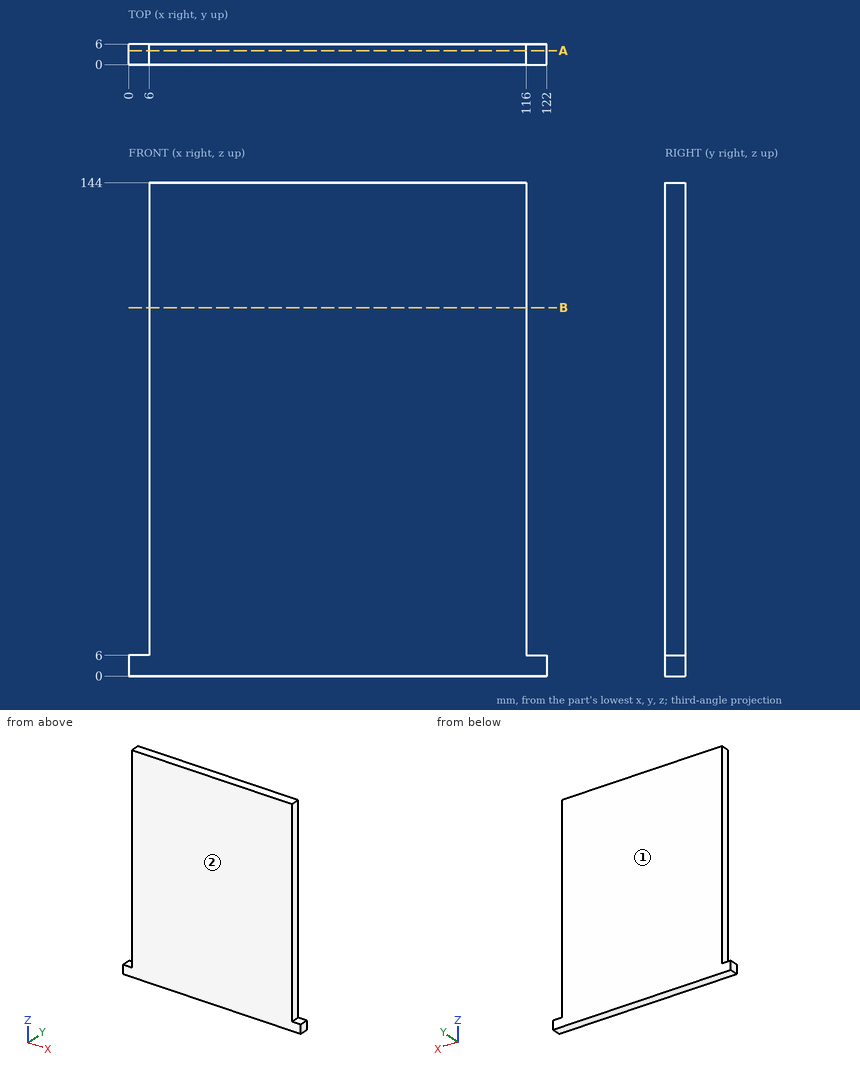
The figure shows three views and two pictorial views of one solid part (mm, origin at its lowest corner). Answer the questions. Round coordinates to 2 decimals unless told otherwise and drop trailing zeros. Write each loop counter-clockwise with the first axis right and the second up, starting at its lowest first coordinate (ties: lowest second). Pieces come first, ordered by that corner, then holes. Notation, with made-up numbers: M 54.5,38 L 101.5,38 A15 ccw 101.5,63 Z; hole C 30.5,-24 d1. An arc over 180 degrees is marked long. Use a Markdown table: item, result.
1) The part is cut by section A-A (y = 4.05). Write down the section's boundary in (x, z), plus the area to 3 significant figures.
Answers follow:
| item | result |
|---|---|
| outline | M 0,0 L 122,0 L 122,6 L 116,6 L 116,144 L 6,144 L 6,6 L 0,6 Z |
| area | 15,900 mm2 |
2) The part is cut by section B-B (z = 107.5). Write down the section's boundary in (x, y).
Answers follow:
| item | result |
|---|---|
| outline | M 6,0 L 116,0 L 116,6 L 6,6 Z |
3) For a pull along Y with two mould halves and no side action, classify the marked faces 1 and 2 as pulls with the +Y half, pulls with the -Y half, needs draft (parallel to the pull), parting line crosses it, or undercut.
Answers follow:
| item | result |
|---|---|
| face 1 | pulls with the +Y half |
| face 2 | pulls with the -Y half |
4) A straight line is drawn through the part: line 1 along X through (y, z) = (5.5, 76). Find the intervals that lie inside material, in ascending order. Write a range as [from, to].
Answers follow:
| item | result |
|---|---|
| line 1 | x = [6, 116] |
5) Flat-ended cylindrical pins translate along their axes: pin 1 (1.8 mm diameter, centred on x = 2.5, y = 2.5, fed in from +Z); pin 2 (3 mm diameter, centred on x = 42.5, y = 3, fed in from -Z); pin 3 (1.8 mm diameter, centred on y = 3, z = 88.5, fed in from +X); pin 4 (1.8 mm diameter, centred on y = 3, z = 63, fed in from -X). Find the tip coordinate at first contact, or state that the pin passes through.
Answers follow:
| item | result |
|---|---|
| pin 1 | stops at z = 6 |
| pin 2 | stops at z = 0 |
| pin 3 | stops at x = 116 |
| pin 4 | stops at x = 6 |
